```python
from build123d import *

# Parameters (mm, degrees)
SKETCH1_W           = 30
SKETCH1_H           = 36
BOSS_EXTRUDE1_DEPTH = 2
SKETCH2_W           = 11
SKETCH2_H           = 4
SKETCH2_W_2         = 6
SKETCH2_R           = 1.5
CUT_EXTRUDE2_DEPTH  = 10


with BuildPart() as part:
    # Sketch1 → Boss-Extrude1 (new body)
    with BuildSketch(Plane(origin=(0, 0, 0), x_dir=(0, 0, -1), z_dir=(1, 0, 0))):
        Rectangle(SKETCH1_W, SKETCH1_H)
    extrude(amount=BOSS_EXTRUDE1_DEPTH)

    # Sketch2 → Cut-Extrude2 (cut)
    with BuildSketch(Plane(origin=(2, 0, 0), x_dir=(0, 0, -1), z_dir=(1, 0, 0))):
        with Locations((0, 4.75)):
            Rectangle(SKETCH2_W, SKETCH2_H)
        with Locations((-2.5, -4.75)):
            Rectangle(SKETCH2_W_2, SKETCH2_H)
        with Locations((2.5, -3.75)):
            Circle(SKETCH2_R)
    extrude(amount=-CUT_EXTRUDE2_DEPTH, mode=Mode.SUBTRACT)


solid = part.part
```
The listing builds one solid part. Answer for the finished solid, in the listing's coordinates (mm). A direction names the side the tool comes from. Coordinates: 2 decimals unless noted, no trailing zeros. Order: outer loops, then holes, each group sorted by start corner. A loop starts at its lowest first (then second) coordinate and runs counter-clockwise, first axis right, second up. Notation, with made-up numbers: M 65.25,15 L 86.25,15 A23 cw 86.25,28 Z; hole C 41.5,-23.75 d6. An arc over 180 degrees is marked long. Answer as a JSON object with one key per item and string values. Group by question number.
1. A tool of negligible diameter and unlimited length cuts with its end or side. For faces 5 (the flat face through (1, 0, 15)), 6 (the flat face through (1, -6.75, 3)), from which of +Z, -Z, +X, -X, +Y, -Y can it reach the whole face along a straight path? Write none if from no direction.
2. Determine the mould class of faces 1 (the flat face through (0, 0, 0)), 2 (the flat face through (1, 5, 5.5)), 3 (the flat face through (1, 18, 0)), 4 (the flat face through (1, -5, 5.5)) for opening direction Y: released by +Y, released by -Y, zero draft, split by the parting line, or undercut.
3. A flat-ended cylindrical pin translates along its axis: P1, Ø1.8, axis at y = -3.75, z = -2.5, coming from the -X side. Find the tip coordinate at first contact, or state that the pin passes through.
4. Section B-B on y = -3.75 is taken. Write down the section's boundary in (x, z), then the cut area to 3 significant figures.
5. Straight lines are drawn through the part: line 1 (Y direction, x = 1.6, z = -2.5); line 2 (Y direction, x = 0.8, z = 2.5); line 3 (Z direction, x = 1, y = -4.5). For each, find the intervals that lie inside material, in ascending order.
6. Section C-C on x = 0.7 is taken. Write down the section's boundary in (y, z), then the cut area to 3 significant figures.
7. Section A-A on z = -2.5 is taken. Write down the section's boundary in (x, y), then the cut area to 3 significant figures.
Values follow:
{
 "1": {"face 5": "+Z, +X, -X, +Y, -Y", "face 6": "+X, -X"},
 "2": {"face 1": "zero draft", "face 2": "undercut", "face 3": "released by +Y", "face 4": "undercut"},
 "3": {"P1": "through"},
 "4": {"outline": "M 0,-15 L 2,-15 L 2,-4 L 0,-4 Z; M 0,-1 L 2,-1 L 2,-0.5 L 0,-0.5 Z; M 0,5.5 L 2,5.5 L 2,15 L 0,15 Z", "area": "42.0 mm2"},
 "5": {"line 1": "-18 to -5.25, -2.25 to 2.75, 6.75 to 18", "line 2": "-18 to -6.75, -2.75 to 2.75, 6.75 to 18", "line 3": "-15 to -3.8, -1.2 to -0.5, 5.5 to 15"},
 "6": {"outline": "M -18,-15 L 18,-15 L 18,15 L -18,15 Z; hole M -6.75,-0.5 L -2.75,-0.5 L -2.75,5.5 L -6.75,5.5 Z; hole C -3.75,-2.5 d3; hole M 2.75,-5.5 L 6.75,-5.5 L 6.75,5.5 L 2.75,5.5 Z", "area": "1,000 mm2"},
 "7": {"outline": "M 0,-18 L 2,-18 L 2,-5.25 L 0,-5.25 Z; M 0,-2.25 L 2,-2.25 L 2,2.75 L 0,2.75 Z; M 0,6.75 L 2,6.75 L 2,18 L 0,18 Z", "area": "58.0 mm2"}
}
